Read the model definition and answer for the solid it produces. Units are mm, in the model's axes. Face numbers are marked on the shaded views. Give positions to 0.01 mm unless a question says otherwise; leave off trailing zeros. Order: outer loops, then holes, each group sorted by start corner. A loop starts at its lowest first (then second) coordinate and runs counter-clockwise, first axis right, second up. Notation, with made-up numbers: (79, 79) - (134, 79) arc R20 ccw to (134, 97) - close; hole circle Ø4 at (-9.75, 89). An arc over 180 degrees is marked (long way). Return JSON: item names as keys, results as strings.
```python
from build123d import *

# Parameters (mm, degrees)
F_0_1MM_FIT_FOR_POT_R = 10.5
BOSS_EXTRUDE1_DEPTH   = 2.75
SKETCH4_R             = 10.5
SKETCH4_R_2           = 8.25
BOSS_EXTRUDE2_DEPTH   = 4.25
BOSS_EXTRUDE3_DEPTH   = 2
FILLET1_R             = 0.25
BOSS_EXTRUDE4_DEPTH   = 2


with BuildPart() as part:
    # 0.1mm fit for pot → Boss-Extrude1 (new body)
    with BuildSketch(Plane(origin=(0, 0, 0), x_dir=(1, 0, 0), z_dir=(0, 1, 0))):
        Circle(F_0_1MM_FIT_FOR_POT_R)
    extrude(amount=BOSS_EXTRUDE1_DEPTH)

    # Sketch4 → Boss-Extrude2 (add)
    with BuildSketch(Plane(origin=(0, 2.75, 0), x_dir=(1, 0, 0), z_dir=(0, 1, 0))):
        Circle(SKETCH4_R)
        Circle(SKETCH4_R_2, mode=Mode.SUBTRACT)
    extrude(amount=BOSS_EXTRUDE2_DEPTH)

    # Sketch5 → Boss-Extrude3 (add)
    with BuildSketch(Plane(origin=(0, 2.75, 0), x_dir=(1, 0, 0), z_dir=(0, 1, 0))):
        with BuildLine():
            Line((-1, -8.189169677), (-1, -7.05))
            Line((-1, -7.05), (1, -7.05))
            Line((1, -7.05), (1, -8.189169677))
            ThreePointArc((1, -8.189169677), (0, -8.25), (-1, -8.189169677))
        make_face()
    extrude(amount=BOSS_EXTRUDE3_DEPTH)

    # Fillet1
    fillet1_edges = [part.edges().sort_by_distance(p)[0] for p in [
        (1, 3.75, 7.05),
        (-1, 3.75, 7.05),
        (0, 4.75, 7.05),
        (-1, 4.75, 7.619584839),
        (1, 4.75, 7.619584839),
    ]]
    fillet(fillet1_edges, radius=FILLET1_R)

    # Sketch6 → Boss-Extrude4 (add)
    with BuildSketch(Plane.XZ):
        with BuildLine():
            Line((-4.75, 9.3641604), (-4.75, 65))
            Line((-4.75, 65), (4.75, 65))
            Line((4.75, 65), (4.75, 9.3641604))
            ThreePointArc((4.75, 9.3641604), (0, 10.5), (-4.75, 9.3641604))
        make_face()
    extrude(amount=-BOSS_EXTRUDE4_DEPTH)


solid = part.part
```
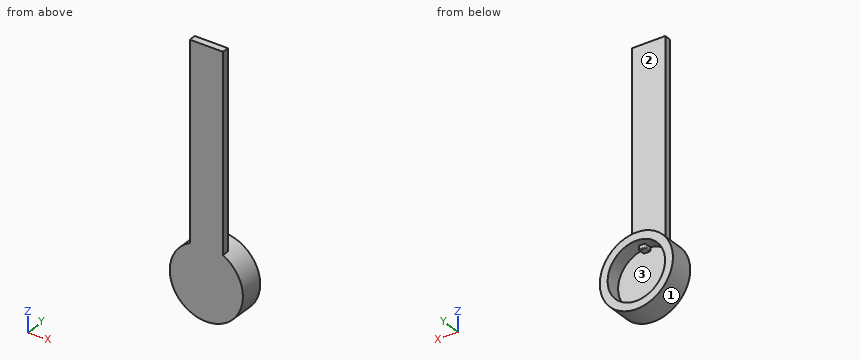
Q1. A cutting plane is placed at D-D (x = -7.25). Write down the section's boundary in (y, z).
Values:
{"outline": "(0, -7.6) - (7, -7.6) - (7, -3.94) - (2.75, -3.94) - (2.75, 3.94) - (7, 3.94) - (7, 7.6) - (0, 7.6) - close"}
Q2. Given pin 1 (1 mm diameter, centred on x = -1.5, z = 55.5, fed in from +Y); pin 2 (1.6 mm diameter, centred on y = 1, z = 44, fed in from +X); pin 3 (1 mm diameter, centred on y = 4, z = 7.5, fed in from +X), each flat-ended and moving along its own axis, determine where each tip first touches the part or whether it passes through.
Values:
{"pin 1": "stops at y = 2", "pin 2": "stops at x = 4.75", "pin 3": "stops at x = 7.83"}
Q3. A cutting plane is placed at B-B (z = 0). Write down the section's boundary in (x, y).
Values:
{"outline": "(-10.5, 0) - (10.5, 0) - (10.5, 7) - (8.25, 7) - (8.25, 2.75) - (-8.25, 2.75) - (-8.25, 7) - (-10.5, 7) - close"}
Q4. A cutting plane is placed at C-C (y = 1.25). Write down the section's boundary in (x, z), and give its area (3 significant figures).
Values:
{"outline": "(-4.75, 9.36) arc R10.5 ccw (long way) to (4.75, 9.36) - (4.75, 65) - (-4.75, 65) - close", "area": "868 mm²"}
Q5. Consider L1, parallel to Z at x = 0, y = 4; L2, parallel to X at y = 3.7, z = 0. Determine where each line is inside the solid, lowest interval first.
Values:
{"L1": "z = -10.5 to -8.25, 7.05 to 10.5", "L2": "x = -10.5 to -8.25, 8.25 to 10.5"}
Q6. A cutting plane is placed at A-A (x = 0). Write down the section's boundary in (y, z).
Values:
{"outline": "(0, -10.5) - (7, -10.5) - (7, -8.25) - (2.75, -8.25) - (2.75, 7.05) - (4.5, 7.05) arc R0.25 ccw to (4.75, 7.3) - (4.75, 8.25) - (7, 8.25) - (7, 10.5) - (2, 10.5) - (2, 65) - (0, 65) - close"}
Q7. Determine the mould class of the marked faces 1, 2 and 3 for opening direction X: released by +X, released by -X, zero draft, split by the parting line, or undercut.
Values:
{"face 1": "split by the parting line", "face 2": "zero draft", "face 3": "undercut"}
